from build123d import *

# Parameters (mm, degrees)
F1_DEPTH = 200
F3_R     = 16.7976843787
F4_DEPTH = 430
F6_W     = 175.9967375547
F6_H     = 67.8384676576
F7_DEPTH = 100
F9_DEPTH = 175


with BuildPart() as f1:
    # F0 (on Front) → F1 (new body)
    with BuildSketch(Plane.XZ):
        with BuildLine():
            add(Edge.make_bspline(
                [(-23.6778533361, 19.5495877862), (-32.3621949462, -21.3626975394), (-12.9401370946, -43.7215901911)],
                knots=[1.1743261985, 1.1743261985, 1.1743261985, 2.6132353561, 2.6132353561, 2.6132353561], degree=2, weights=[1, 0.7521652597, 1]))
            Line((-12.9401370946, -43.7215901911), (12.9401370946, -43.7215901911))
            add(Edge.make_bspline(
                [(12.9401370946, -43.7215901911), (32.3621949462, -21.3626975394), (23.6778533361, 19.5495877862)],
                knots=[3.6699499511, 3.6699499511, 3.6699499511, 5.1088591087, 5.1088591087, 5.1088591087], degree=2, weights=[1, 0.7521652597, 1]))
            Line((23.6778533361, 19.5495877862), (-23.6778533361, 19.5495877862))
        make_face()
    extrude(amount=F1_DEPTH)

    # F3 (on offset) → F4 (join)
    with BuildSketch(Plane.XZ.offset(-230)):
        with Locations((0, 19.52576451)):
            Circle(F3_R)
    extrude(amount=F4_DEPTH)

    # F6 (on offset) → F7 (cut)
    with BuildSketch(Plane.YZ.offset(-30)):
        with Locations((-99.9427214265, -43.750282377)):
            Rectangle(F6_W, F6_H)
    extrude(amount=F7_DEPTH, mode=Mode.SUBTRACT)

    # F8 (on face) → F9 (join)
    with BuildSketch(Plane.XZ.offset(11.9443526492)):
        with BuildLine():
            ThreePointArc((-23.9079126368, -18.4283503945), (-21.4691661744, -95.1354199868), (44.5844215941, -56.0605488718))
            ThreePointArc((44.5844215941, -56.0605488718), (39.0748711148, -34.591382697), (23.907912636, -18.428350394))
            add(Edge.make_bspline(
                [(23.907912636, -18.428350394), (23.7403211383, -19.2740561298), (23.5629806702, -20.1178270573), (23.375722619, -20.959489825), (23.1783610081, -21.7988580379), (22.9706905105, -22.6357318329), (22.7524836933, -23.4698972976), (22.5234871985, -24.301125666), (21.8162555534, -26.7404941038), (21.3073183679, -28.3392219433), (20.754454425, -29.9239250097), (20.1551733117, -31.4923659659), (19.5066312989, -33.0414940382), (18.8054862218, -34.5673766033), (18.0477798353, -36.0651478958), (16.7672298185, -38.3517175377), (16.2868400055, -39.1637140236), (15.7860476096, -39.9635970623), (15.2638749499, -40.7499882648), (14.7193047849, -41.5211878034), (14.1512732931, -42.2751690498), (13.5586431482, -43.0095590272), (12.9401370946, -43.7215901911)],
                knots=[0.2378023461, 0.2378023461, 0.2378023461, 0.2378023461, 0.2378023461, 0.2378023461, 0.2378023461, 0.2378023461, 0.2378023461, 0.4264523686, 0.4264523686, 0.4264523686, 0.4264523686, 0.4264523686, 0.4264523686, 0.4264523686, 0.7935523887, 0.7935523887, 0.7935523887, 0.7935523887, 0.7935523887, 0.7935523887, 0.7935523887, 1, 1, 1, 1, 1, 1, 1, 1, 1], degree=8))
            Line((12.9401370946, -43.7215901911), (-12.9401370946, -43.7215901911))
            add(Edge.make_bspline(
                [(-12.9401370946, -43.7215901911), (-13.5586431482, -43.0095590272), (-14.1512732931, -42.2751690498), (-14.7193047849, -41.5211878034), (-15.2638749499, -40.7499882648), (-15.7860476096, -39.9635970623), (-16.2868400055, -39.1637140236), (-16.7672298185, -38.3517175377), (-18.043616681, -36.0725816877), (-18.7977894386, -34.5825873298), (-19.4959463044, -33.0647358798), (-20.1419918652, -31.5238279251), (-20.7392245037, -29.9637460227), (-21.2904531713, -28.3875056791), (-21.7981390661, -26.7973221406), (-22.507625983, -24.3586134522), (-22.739531347, -23.5193487447), (-22.9604201458, -22.6770764585), (-23.17055429, -21.8320330534), (-23.3701686358, -20.9844394656), (-23.5594750148, -20.1345019592), (-23.7386651299, -19.2824127385), (-23.9079126368, -18.4283503945)],
                knots=[0, 0, 0, 0, 0, 0, 0, 0, 0, 0.2064476064, 0.2064476064, 0.2064476064, 0.2064476064, 0.2064476064, 0.2064476064, 0.2064476064, 0.5716829759, 0.5716829759, 0.5716829759, 0.5716829759, 0.5716829759, 0.5716829759, 0.5716829759, 0.7621973133, 0.7621973133, 0.7621973133, 0.7621973133, 0.7621973133, 0.7621973133, 0.7621973133, 0.7621973133, 0.7621973133], degree=8))
        make_face()
        with BuildLine():
            add(Edge.make_bspline(
                [(23.907912636, -18.428350394), (23.7403211383, -19.2740561298), (23.5629806702, -20.1178270573), (23.375722619, -20.959489825), (23.1783610081, -21.7988580379), (22.9706905105, -22.6357318329), (22.7524836933, -23.4698972976), (22.5234871985, -24.301125666), (21.8162555534, -26.7404941038), (21.3073183679, -28.3392219433), (20.754454425, -29.9239250097), (20.1551733117, -31.4923659659), (19.5066312989, -33.0414940382), (18.8054862218, -34.5673766033), (18.0477798353, -36.0651478958), (16.7672298185, -38.3517175377), (16.2868400055, -39.1637140236), (15.7860476096, -39.9635970623), (15.2638749499, -40.7499882648), (14.7193047849, -41.5211878034), (14.1512732931, -42.2751690498), (13.5586431482, -43.0095590272), (12.9401370946, -43.7215901911)],
                knots=[0.2378023461, 0.2378023461, 0.2378023461, 0.2378023461, 0.2378023461, 0.2378023461, 0.2378023461, 0.2378023461, 0.2378023461, 0.4264523686, 0.4264523686, 0.4264523686, 0.4264523686, 0.4264523686, 0.4264523686, 0.4264523686, 0.7935523887, 0.7935523887, 0.7935523887, 0.7935523887, 0.7935523887, 0.7935523887, 0.7935523887, 1, 1, 1, 1, 1, 1, 1, 1, 1], degree=8))
            ThreePointArc((23.907912636, -18.428350394), (-5e-10, -11.4761272777), (-23.9079126368, -18.4283503945))
            add(Edge.make_bspline(
                [(-12.9401370946, -43.7215901911), (-13.5586431482, -43.0095590272), (-14.1512732931, -42.2751690498), (-14.7193047849, -41.5211878034), (-15.2638749499, -40.7499882648), (-15.7860476096, -39.9635970623), (-16.2868400055, -39.1637140236), (-16.7672298185, -38.3517175377), (-18.043616681, -36.0725816877), (-18.7977894386, -34.5825873298), (-19.4959463044, -33.0647358798), (-20.1419918652, -31.5238279251), (-20.7392245037, -29.9637460227), (-21.2904531713, -28.3875056791), (-21.7981390661, -26.7973221406), (-22.507625983, -24.3586134522), (-22.739531347, -23.5193487447), (-22.9604201458, -22.6770764585), (-23.17055429, -21.8320330534), (-23.3701686358, -20.9844394656), (-23.5594750148, -20.1345019592), (-23.7386651299, -19.2824127385), (-23.9079126368, -18.4283503945)],
                knots=[0, 0, 0, 0, 0, 0, 0, 0, 0, 0.2064476064, 0.2064476064, 0.2064476064, 0.2064476064, 0.2064476064, 0.2064476064, 0.2064476064, 0.5716829759, 0.5716829759, 0.5716829759, 0.5716829759, 0.5716829759, 0.5716829759, 0.5716829759, 0.7621973133, 0.7621973133, 0.7621973133, 0.7621973133, 0.7621973133, 0.7621973133, 0.7621973133, 0.7621973133, 0.7621973133], degree=8))
            Line((-12.9401370946, -43.7215901911), (12.9401370946, -43.7215901911))
        make_face()
    extrude(amount=F9_DEPTH)


solid = f1.part
Design review of the part built by this model. Coordinates are the model's own, in mm. A direction names the side the tool comes from. Round coordinates to 2 decimals unless told otherwise and drop trailing zeros. Loops run counter-clockwise (first coordinate to the right, second up) from the corner with the lowest first, then second, coordinate; pieces in that order, holes last. Notation, with made-up numbers: (-19, 87) -> (34, 87) arc R25 ccw to (34, 118) -> close; hole circle Ø4 at (73.5, 59.5). An arc over 180 degrees is marked (long way). Use one line per item in the form item = value. Start each with the question number.
Q1. We need section B-B on y = 116.5. Give the boundary of the cut face in (x, z).
Q2. We need section A-A on x = 0. Give the boundary of the cut face in (y, z).
Q3. Draft analysis for pull direction Y (two halves, no side actions). For faces 6 (the face through (0, -11.944, -11)), 7 (the face through (0, 230, 20)), 8 (the face through (0, -6, -43.722)), state which applies: +Y half, -Y half, draft (parallel to the pull), parting line (faces both ways), or undercut.
Q4. Wall thickness on line 1 along Y through (x, z) = (-23, -91.5); line 2 along Z through (x, y) = (-7.5, -121.5); line 3 along Z through (x, y) = (6, -86): over which ranges is each line inside the solid? List them lowest first. Write a range as [from, to].
Q5. Machinability: for faces 1 (the face through (0, -101, -9.831)), 2 (the face through (0, -194, -43.722)), 3 (the face through (0, -200, -3)), 4 (the face through (-2.19, 65.79, 36.18)), 5 (the face through (-1, -186.944, -55)), which of the approach directions +Z, -Z, +X, -X, +Y, -Y give a long, thin tool a straight path to every point of the face, cutting with its end or side? Answer none if there is none.
Q6. For pin 1 Ø5 at (x, y) = (29, -71.5) entering from -Z; pin 2 Ø1 at (x, y) = (34, -61.5) entering from -Z; pin 3 Ø4 at (x, y) = (-23.5, -27.5) entering from +Z, all flat-tipped, find the tip position at first contact; note any pin that passes through.
Q7. We need section C-C on z = 27.5. Give the boundary of the cut face in (x, y), then the cut area to 3 significant figures.
Calculated:
q1.outline = circle Ø33.6 at (0, 19.53)
q2.outline = (-200, -43.72) -> (-187.94, -43.72) -> (-187.94, -9.83) -> (-11.94, -9.83) -> (-11.94, -11.48) -> (-186.94, -11.48) -> (-186.94, -100.64) -> (-11.94, -100.64) -> (-11.94, -43.72) -> (0, -43.72) -> (0, 2.73) -> (230, 2.73) -> (230, 36.32) -> (-200, 36.32) -> close
q3.face_6 = undercut
q3.face_7 = +Y half
q3.face_8 = draft
q4.line_1 = [-186.94, -11.94]
q4.line_2 = [-100.01, -12.11], [-9.83, 34.56]
q4.line_3 = [-100.24, -11.88], [-9.83, 35.22]
q5.face_1 = +X, -X
q5.face_2 = -Z, +X, -X, -Y
q5.face_3 = +Z, -Z, +X, -X, -Y
q5.face_4 = +Y
q5.face_5 = -Z, +X, -X
q6.pin_1 = -91.91
q6.pin_2 = -85.48
q6.pin_3 = 19.55
q7.outline = (-14.78, -200) -> (14.78, -200) -> (14.78, 230) -> (-14.78, 230) -> close
q7.area = 12,700 mm²
